Geometry check sheet. Reference: drawing and pictorial views, mm from the part's lowest x, y, z. Round coordinates to 2 decimals unless told otherwise and drop trailing zeros. Write each loop counter-clockwise with the first axis right and the second up, starting at its lowest first coordinate (ties: lowest second). Pieces come first, ordered by that corner, then holes. Notation, with made-up numbers: M -4.5,88.5 L 52.5,88.5 A17 cw 52.5,106.5 Z; hole C 1,-20 d8. An arc over 180 degrees is marked long. Answer in a Markdown table with one row per item. Add a question column.
1. Sectioned sample at C-C on y = 1.55. Count the separate pieces of the cut face and the enclosed holes in it, plus the area to 3 significant figures.
2. Sectioned sample at B-B on z = 37. Record the cut outline in (x, y), plus the area to 3 significant figures.
3. Sectioned sample at D-D on z = 67.5. Record the cut outline in (x, y).
4. Sectioned sample at A-A on x = 144. Record the cut outline in (y, z).
5. Material ranges on probe 1 along X at (y, z) = (3.15, 138); probe 2 along X at (y, z) = (2.35, 20.5); probe 3 along Z at (x, y) = (144, 1.3), recorded low to high.
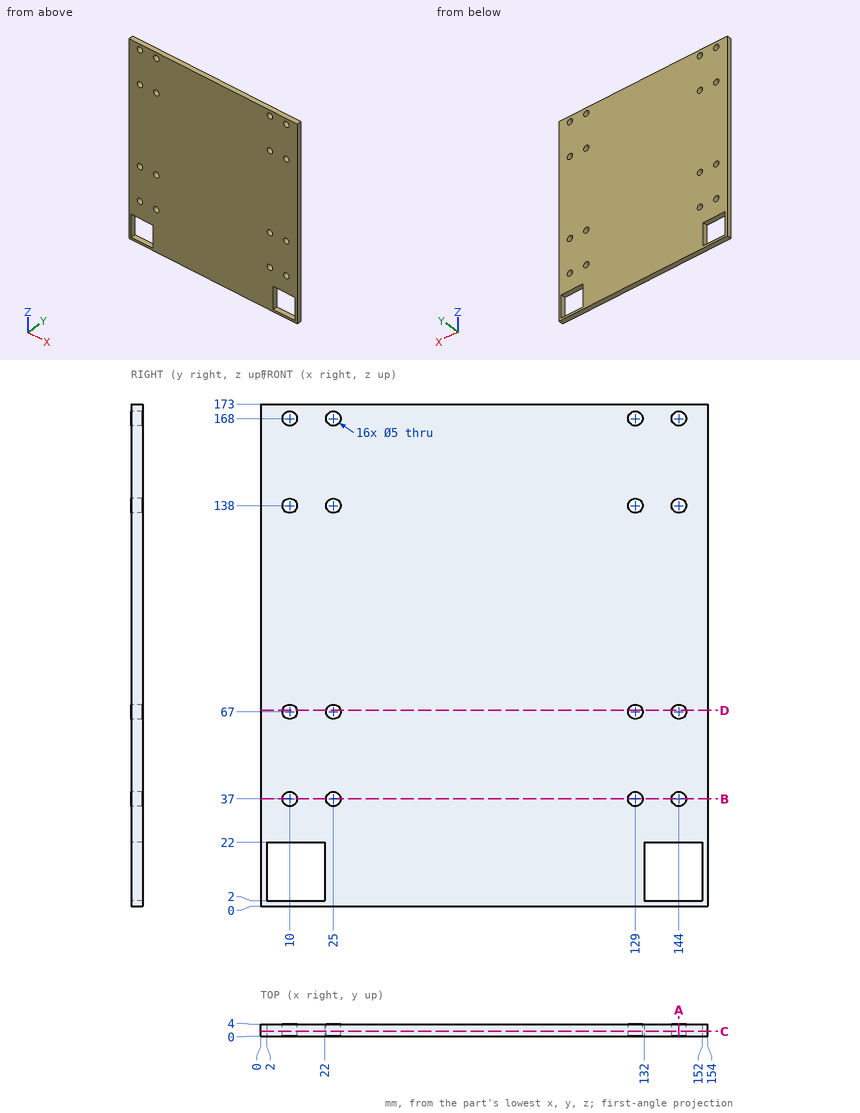
Geometry check:
| question | item | result |
|---|---|---|
| 1 | separate pieces | 1 |
| 1 | enclosed holes | 18 |
| 1 | area | 25,500 mm2 |
| 2 | outline | M 0,0 L 7.5,0 L 7.5,4 L 0,4 Z; M 12.5,0 L 22.5,0 L 22.5,4 L 12.5,4 Z; M 27.5,0 L 126.5,0 L 126.5,4 L 27.5,4 Z; M 131.5,0 L 141.5,0 L 141.5,4 L 131.5,4 Z; M 146.5,0 L 154,0 L 154,4 L 146.5,4 Z |
| 2 | area | 536 mm2 |
| 3 | outline | M 0,0 L 7.55,0 L 7.55,4 L 0,4 Z; M 12.45,0 L 22.55,0 L 22.55,4 L 12.45,4 Z; M 27.45,0 L 126.55,0 L 126.55,4 L 27.45,4 Z; M 131.45,0 L 141.55,0 L 141.55,4 L 131.45,4 Z; M 146.45,0 L 154,0 L 154,4 L 146.45,4 Z |
| 4 | outline | M 0,0 L 4,0 L 4,2 L 0,2 Z; M 0,22 L 4,22 L 4,34.5 L 0,34.5 Z; M 0,39.5 L 4,39.5 L 4,64.5 L 0,64.5 Z; M 0,69.5 L 4,69.5 L 4,135.5 L 0,135.5 Z; M 0,140.5 L 4,140.5 L 4,165.5 L 0,165.5 Z; M 0,170.5 L 4,170.5 L 4,173 L 0,173 Z |
| 5 | probe 1 | x = 0 to 7.5, 12.5 to 22.5, 27.5 to 126.5, 131.5 to 141.5, 146.5 to 154 |
| 5 | probe 2 | x = 0 to 2, 22 to 132, 152 to 154 |
| 5 | probe 3 | z = 0 to 2, 22 to 34.5, 39.5 to 64.5, 69.5 to 135.5, 140.5 to 165.5, 170.5 to 173 |
